Could you check a few things on this drawing? It's one solid part, dimensions in mm from its lowest x, y, z. A direction names the side the tool comes from. Round coordinates to 2 decimals unless told otherwise and drop trailing zeros. Write each loop counter-clockwise with the first axis right and the second up, starting at its lowest first coordinate (ties: lowest second). Pieces come first, ordered by that corner, then holes. Notation, with made-up numbers: (71.25, 71) - (97.25, 71) arc R33 cw to (97.25, 104) - close; hole circle Ø5 at (24.5, -24). An arc over 180 degrees is marked (long way). Put each result on its own line as item: value.
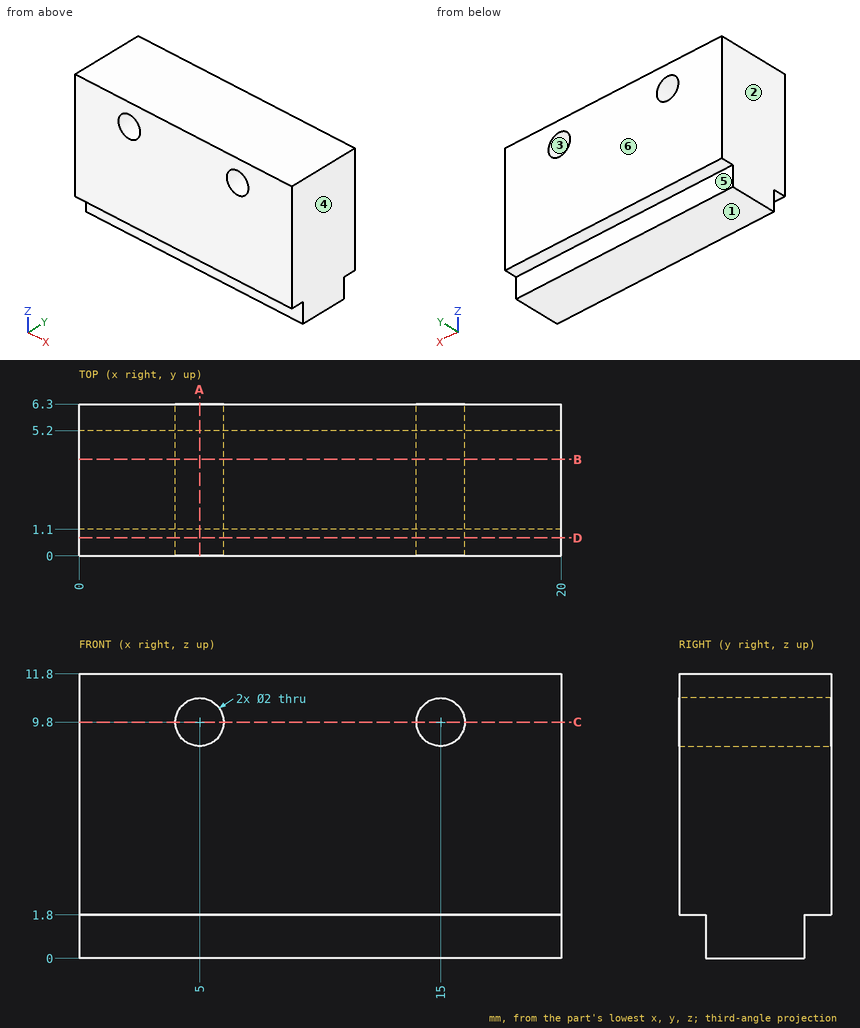
(1) For the marked faces 5 and 6, which set-ups out of +Z, -Z, +X, -X, +Y, -Y let a thin tool reach every point of the face, with its end or its side?
Values found:
face 5: -Z, +X, -X, +Y
face 6: +Z, -Z, +X, -X, +Y
(2) Please list where these lines run through material, in increasing order: probe 1 along X at (y, z) = (5, 9.8); probe 2 along Y at (x, z) = (11, 1.5); probe 3 along Z at (x, y) = (13, 6). Write a range as from..to.
Values found:
probe 1: x = 0..4, 6..14, 16..20
probe 2: y = 1.1..5.2
probe 3: z = 1.8..11.8
(3) Imagine slicing it at C-C, the plane z = 9.8. List the corners of the cut face in (x, y) for me, then the cut area to 3 significant figures.
Values found:
outline: (0, 0) - (4, 0) - (4, 6.3) - (0, 6.3) - close; (6, 0) - (14, 0) - (14, 6.3) - (6, 6.3) - close; (16, 0) - (20, 0) - (20, 6.3) - (16, 6.3) - close
area: 101 mm^2
(4) Imagine slicing it at D-D, the plane y = 0.75. List the corners of the cut face in (x, z) for me, then the cut area to 3 significant figures.
Values found:
outline: (0, 1.8) - (20, 1.8) - (20, 11.8) - (0, 11.8) - close; hole circle Ø2 at (5, 9.8); hole circle Ø2 at (15, 9.8)
area: 194 mm^2
(5) I'm going to push flat-ended pins straight in: pin 1 (1.4 mm diameter, centred on x = 13.5, z = 1, fed in from -Y); pin 2 (1.4 mm diameter, centred on x = 6, z = 1, fed in from +Y). Where does each tip first touch, or does it pass through?
Values found:
pin 1: stops at y = 1.1
pin 2: stops at y = 5.2
(6) Imagine slicing it at A-A, the plane x = 5. List the corners of the cut face in (y, z) for me, then the cut area to 3 significant figures.
Values found:
outline: (0, 1.8) - (1.1, 1.8) - (1.1, 0) - (5.2, 0) - (5.2, 1.8) - (6.3, 1.8) - (6.3, 8.8) - (0, 8.8) - close; (0, 10.8) - (6.3, 10.8) - (6.3, 11.8) - (0, 11.8) - close
area: 57.8 mm^2
(7) If we mould it in two halves opening along X, with no side actions, what happens to the marked faces 1, 2, 3 and 4? For each: pulls with the +X half, pulls with the -X half, needs draft (parallel to the pull), parting line crosses it, or undercut.
Values found:
face 1: needs draft
face 2: pulls with the -X half
face 3: undercut
face 4: pulls with the +X half
(8) Imagine slicing it at B-B, the plane y = 4. List the corners of the cut face in (x, z) for me.
Values found:
outline: (0, 0) - (20, 0) - (20, 11.8) - (0, 11.8) - close; hole circle Ø2 at (5, 9.8); hole circle Ø2 at (15, 9.8)
